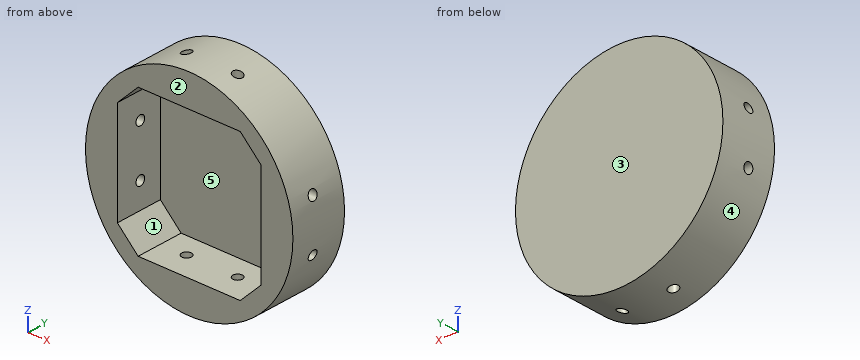
Autodesk Inventor part; units mm, degrees
ref_plane "YZ Plane" through (0, 0, 0) normal (1, 0, 0) x (0, 1, 0)
ref_plane "XZ Plane" through (0, 0, 0) normal (0, 1, 0) x (-1, 0, 0)
ref_plane "XY Plane" through (0, 0, 0) normal (0, 0, 1) x (1, 0, 0)
sketch "Boceto1" plane through (0, 0, 0) normal (0, 1, 0) x (-1, 0, 0)
  circle A0 centre (0, 0) radius 32.5
  line L0 (0, 0) -> (22.5, 0)
  line L1 (22.5, 0) -> (22.5, -16)
  line L2 (22.5, -16) -> (22.5, 16)
  line L3 (0, 0) -> (0, 22.5)
  line L4 (0, 22.5) -> (16, 22.5)
  line L5 (16, 22.5) -> (-16, 22.5)
  line L6 (0, 0) -> (-22.5, 0)
  line L7 (-22.5, 0) -> (-22.5, 16)
  line L8 (-22.5, 16) -> (-22.5, -16)
  line L9 (0, 0) -> (0, -22.5)
  line L10 (0, -22.5) -> (-16, -22.5)
  line L11 (-16, -22.5) -> (16, -22.5)
  line L12 (22.5, 16) -> (16, 22.5)
  line L13 (-16, 22.5) -> (-22.5, 16)
  line L14 (-22.5, -16) -> (-16, -22.5)
  line L15 (16, -22.5) -> (22.5, -16)
  dimension "d0" = 65
  dimension "d1" = 22.5
  dimension "d3" = 16
  dimension "d4" = 32
  dimension "d7" = 360
extrude "Extrusión1" add sketch "Boceto1" along normal blind 15
sketch "Boceto2" plane through (-16, 0, -22.5) normal (0, 0, 1) x (1, 0, 0)
  line L0 (16, 0) -> (16, 8)
  line L1 (16, 8) -> (24, 8)
  line L2 (24, 8) -> (8, 8)
  circle A0 centre (8, 8) radius 1.5
  circle A1 centre (24, 8) radius 1.5
  dimension "d11" = 8
  dimension "d12" = 8
  dimension "d13" = 16
  dimension "d15" = 3
  dimension "d16" = 3
extrude "Extrusión2" cut sketch "Boceto2" along normal mid plane 10200
sketch "Boceto3" plane through (22.5, 0, -16) normal (-1, 0, 0) x (0, 0, 1)
  line L0 (16, 0) -> (16, 8)
  line L1 (16, 8) -> (24, 8)
  line L2 (24, 8) -> (8, 8)
  circle A0 centre (8, 8) radius 1.5
  circle A1 centre (24, 8) radius 1.5
  dimension "d19" = 8
  dimension "d20" = 8
  dimension "d21" = 16
  dimension "d22" = 3
  dimension "d23" = 3
extrude "Extrusión3" cut sketch "Boceto3" against normal mid plane 10200
sketch "Boceto4" plane through (0, 15, 0) normal (0, 1, 0) x (1, 0, 0)
  circle A0 centre (0, 0) radius 32.5
extrude "Extrusión4" add sketch "Boceto4" along normal blind 3
properties part number "acople pinza"
Work out the finished part from the listing and answer in its coordinate system (mm). Face numbers are marked on the shaded views. A direction names the side the tool comes from. Give positions to 0.01 mm unless a question says otherwise; leave off trailing zeros. Order: outer loops, then holes, each group sorted by start corner. A loop starts at its lowest first (then second) coordinate and runs counter-clockwise, first axis right, second up. Notation, with made-up numbers: (-20, 57.5) -> (9, 57.5) arc R24 cw to (9, 83.5) -> close; hole circle Ø8 at (31.25, 45). An arc over 180 degrees is marked (long way). Answer as CSV lines item,"result". Start each with the question number.
(1) Section C-C, the plane y = 5 is taken. Write down the section's boundary in (x, z), plus the area to 3 significant figures.
(2) For a pull along Z with two mould halves and no side action, classify the marked faces 3, 4 and 5 as released by +Z, released by -Z, zero draft, split by the parting line, or undercut.
(3) Consider line 1 along Y through (x, z) = (28.5, 8); line 2 along Z through (x, y) = (-25.25, 8); line 3 along X through (y, z) = (8, 27). Determine where each line is inside the solid, lowest interval first.
(4) Section B-B, the plane z = 26 is taken. Write down the section's boundary in (x, y), plus the area to 3 significant figures.
(5) Each of these flat-tipped pins is pushed along its axis until it touches: pin 1 Ø2 at (y, z) = (16, -6) entering from -X; pin 2 Ø1.8 at (x, y) = (-8, 8) entering from +Z; pin 3 Ø10 at (x, z) = (-6, 24) entering from -Y; pin 4 Ø4 at (y, z) = (8, -8) entering from +X. Where does it stop, or does it pass through?
(6) Which of the six approach directions +Z, -Z, +X, -X, +Y, -Y give full straight-line access (tool end or side, diameter ignored) to the marked faces 1 and 2?
(7) Section D-D, the plane z = 0 is taken. Write down the section's boundary in (x, y).
(8) Section A-A, the plane x = -8 is taken. Write down the section's boundary in (y, z), plus the area to 3 significant figures.
Entries:
1,outline,"circle Ø65 at (0, 0); hole (-22.5, -16) -> (-16, -22.5) -> (16, -22.5) -> (22.5, -16) -> (22.5, 16) -> (16, 22.5) -> (-16, 22.5) -> (-22.5, 16) -> close"
1,area,"1,380 mm²"
2,face 3,"zero draft"
2,face 4,"split by the parting line"
2,face 5,"undercut"
3,line 1,"0 to 6.5, 9.5 to 18"
3,line 2,"-20.46 to -9.5, -6.5 to 6.5, 9.5 to 20.46"
3,line 3,"-18.09 to -9.5, -6.5 to 6.5, 9.5 to 18.09"
4,outline,"(-19.5, 0) -> (19.5, 0) -> (19.5, 18) -> (-19.5, 18) -> close; hole circle Ø3 at (-8, 8); hole circle Ø3 at (8, 8)"
4,area,"688 mm²"
5,pin 1,"x = -32.11"
5,pin 2,"through"
5,pin 3,"y = 0"
5,pin 4,"x = 31.94"
6,face 1,"-Y"
6,face 2,"+Z, -Z, +X, -X, -Y"
7,outline,"(-32.5, 0) -> (-22.5, 0) -> (-22.5, 15) -> (22.5, 15) -> (22.5, 0) -> (32.5, 0) -> (32.5, 18) -> (-32.5, 18) -> close"
8,outline,"(0, -31.5) -> (6.5, -31.5) -> (6.5, -22.5) -> (0, -22.5) -> close; (0, 22.5) -> (6.5, 22.5) -> (6.5, 31.5) -> (0, 31.5) -> close; (9.5, -31.5) -> (18, -31.5) -> (18, 31.5) -> (9.5, 31.5) -> (9.5, 22.5) -> (15, 22.5) -> (15, -22.5) -> (9.5, -22.5) -> close"
8,area,"405 mm²"
